Autodesk Inventor part; units mm, degrees
ref_plane "XZ Plane" through (0, 0, 0) normal (0, 1, 0) x (-1, 0, 0)
ref_plane "XY Plane" through (0, 0, 0) normal (0, 0, 1) x (1, 0, 0)
sketch "Sketch1" plane through (0, 0, 0) normal (0, 1, 0) x (-1, 0, 0)
  line L0 (0, 0) -> (0, -60)
  line L1 (0, 0) -> (-50, 0)
  line L2 (-5, -60) -> (-5, -5)
  line L3 (-5, -5) -> (-50, -5)
  line L4 (-47.5, 69.0442) -> (-47.5, -71.5611) construction
  line L5 (-50, 0) -> (-55, 0)
  line L6 (-55, 0) -> (-55, -50)
  line L7 (-55, -50) -> (-75, -50)
  line L8 (-75, -50) -> (-75, -60)
  line L9 (-75, -60) -> (-45, -60)
  line L10 (-5, -60) -> (-21, -60)
  circle A0 centre (-47.5, -73.124) radius 8.5
  line L11 (16.7028, -43.5) -> (-102.7124, -43.5) construction
  line L12 (-45, -26.5) -> (-50, -26.5)
  line L13 (-50, -26.5) -> (-50, -60.5)
  line L14 (-50, -60.5) -> (-45, -60.5)
  line L15 (-45, -60.5) -> (-45, -26.5)
  line L16 (-45, -43.5) -> (-50, -43.5) construction
  line L17 (-21, -60) -> (-21, -67.124)
  line L18 (-21, -67.124) -> (-30, -67.124)
  line L19 (-39, -67.124) -> (-39, -60)
  line L20 (-39, -60) -> (-45, -60) construction
  line L21 (-15.952, -100.4576) -> (-35.952, -100.4576)
  line L22 (-35.952, -108.4576) -> (-15.952, -108.4576)
  line L23 (-15.952, -108.4576) -> (-15.952, -100.4576)
  line L24 (-15.952, -73.124) -> (-76.4965, -73.124) construction
  line L25 (-30, -57.9879) -> (-30, -83.8601) construction
  line L26 (-25.952, -100.4576) -> (-25.952, -108.4576) construction
  line L27 (-45, -31) -> (-50, -31) construction
  line L28 (-50, -31) -> (-50, -56)
  line L29 (-50, -56) -> (-45, -56) construction
  line L30 (-45, -56) -> (-45, -31)
  line L31 (-45, -56) -> (-50, -56)
  line L32 (-45, -65.1391) -> (-45, -56)
  line L33 (-45, -56) -> (-50, -56)
  line L34 (-50, -56) -> (-50, -65)
  line L35 (-50, -65) -> (-45, -65)
  line L36 (-45, -65) -> (-45, -56)
  arc A1 (-35.952, -108.4576) -> (-35.952, -100.4576) centre (-43.452, -104.4576) ccw
  line L37 (-30, -67.124) -> (-39, -67.124)
  point P0 (-47.5, -43.5)
  point P1 (-30, -73.124)
  dimension "d9" = 17
  dimension "d0" = 60
  dimension "d1" = 50
  dimension "d2" = 5
  dimension "d3" = 47.5
  dimension "d4" = 5
  dimension "d5" = 50
  dimension "d6" = 20
  dimension "d7" = 30
  dimension "d10" = 38.5
  dimension "d11" = 5
  dimension "d12" = 34
  dimension "d13" = 20
  dimension "d14" = 8
  dimension "d57" = 25
  dimension "d58" = 4.5
  dimension "d59" = 5
  dimension "d60" = 9
  dimension "d61" = 17
  dimension "d62" = 9
  dimension "d63" = 9
  dimension "d64" = 9
  dimension "d65" = 6
sketch "Sketch2" plane through (0, 0, 0) normal (0, 1, 0) x (-1, 0, 0)
  line L0 (0, 0) -> (-60, 0)
  line L1 (-60, 0) -> (-60, -55)
  line L2 (-57.5, -60) -> (0, -60)
  line L3 (0, -60) -> (0, 0)
  line L4 (-5, -60) -> (-21, -60)
  line L5 (-30, -67.124) -> (-39, -67.124)
  line L6 (-57.5, -67.124) -> (-72, -67.124)
  line L7 (-72, -67.124) -> (-72, -59.124)
  line L8 (-72, -59.124) -> (-60, -59.124)
  line L9 (-60, -59.124) -> (-60, 0)
  line L10 (-57.5, -67.124) -> (-57.5, -60)
  point P0 (-60, -67.124)
  dimension "d16" = 57.5
  dimension "d73" = 8
  dimension "d76" = 12
  dimension "d77" = 60
extrude "Extrusion1" add sketch "Sketch2" along normal blind 20
sketch "Sketch3" plane through (0, 20, 0) normal (0, 1, 0) x (1, 0, 0)
  line L0 (5, 5) -> (55, 5)
  line L1 (55, 5) -> (55, 55)
  line L2 (55, 55) -> (5, 55)
  line L3 (5, 55) -> (5, 5)
  line L4 (0, 0) -> (60, 0)
  line L5 (0, 60) -> (0, 0)
  dimension "d23" = 5
  dimension "d24" = 5
  dimension "d25" = 50
  dimension "d26" = 50
extrude "Extrusion2" cut sketch "Sketch3" against normal blind 10
sketch "Sketch5" plane through (0, 0, 0) normal (0, -1, 0) x (1, 0, 0)
  line L0 (57.5, -60) -> (0, -60)
  line L1 (45, -60.5) -> (45, -26.5)
  line L2 (5, -60) -> (5, -5)
  line L3 (50, -26.5) -> (50, -60.5)
  line L4 (45, -26.5) -> (50, -26.5)
  line L5 (50, -60.5) -> (45, -60.5)
  line L6 (52, -60) -> (52, -24.5)
  line L7 (52, -24.5) -> (43, -24.5)
  line L8 (43, -24.5) -> (43, -60)
  line L9 (52, -60.5) -> (52, -60)
  line L10 (52, -60) -> (43, -60)
  point P0 (80, -60)
  dimension "d30" = 40
  dimension "d31" = 2
extrude "Extrusion3" cut sketch "Sketch5" against normal through all contours L0 L3 L4 L1 L8 L7 L6 | L0 L1 L4 L3
sketch "Sketch6" plane through (0, 0, 0) normal (0, 0, 1) x (1, 0, 0)
  line L0 (0, 20) -> (60, 20)
  line L1 (47.5, 0) -> (47.5, 20) construction
  circle A0 centre (47.5, 10) radius 7
  point P0 (47.5, 0)
  dimension "d34" = 14
extrude "Extrusion4" add sketch "Sketch6" along normal blind 25
ref_plane "Work Plane1" through (54.5, 10, 0) normal (1, 0, 0) x (0, 1, 0)
sketch "Sketch7" plane through (54.5, 10, 0) normal (1, 0, 0) x (0, 1, 0)
  line L0 (7, 25) -> (-7, 25)
  line L1 (0, 25) -> (0, 0) construction
  point P0 (-10, 0)
  point P1 (0, 17)
  dimension "d37" = 8
hole "Hole1" at (54.5, 10, 17) direction (-1, 0, 0) diameter 5 end through all
sketch "Sketch8" plane through (0, 10, 0) normal (0, 1, 0) x (1, 0, 0)
  line L0 (36, 11.5) -> (39, 11.5)
  line L1 (39, 11.5) -> (39, 43.5)
  line L2 (39, 43.5) -> (36, 43.5)
  line L3 (36, 43.5) -> (36, 11.5)
  line L4 (45, 60.5) -> (45, 26.5)
  line L5 (-16.7028, 43.5) -> (102.7124, 43.5) construction
  point P0 (0, 0)
  point P1 (47.5, 43.5)
  dimension "d45" = 6
  dimension "d46" = 32
  dimension "d47" = 3
extrude "Extrusion5" cut sketch "Sketch8" against normal blind 4
sketch "Sketch9" plane through (0, 10, 0) normal (0, 1, 0) x (1, 0, 0)
  line L0 (36, 43.5) -> (39, 43.5)
  line L1 (5, 5) -> (5, 55)
  line L2 (8, 18.5) -> (5, 18.5)
  line L3 (5, 18.5) -> (5, 38.5)
  line L4 (5, 38.5) -> (8, 38.5)
  line L5 (8, 38.5) -> (8, 18.5)
  point P0 (0, 0)
  dimension "d50" = 3
  dimension "d51" = 5
  dimension "d52" = 20
extrude "Extrusion6" add sketch "Sketch9" along normal up to surface (10 mm away)
fillet "Fillet1" radius 0.6 4 edges at (5, 15, -38.5) (8, 15, -38.5) (8, 15, -18.5) (5, 15, -18.5)
fillet "Fillet2" radius 1 2 edges at (43, 5, -24.5) (52, 5, -24.5)
sketch "Sketch10" plane through (0, 0, 0) normal (0, -1, 0) x (1, 0, 0)
  line L0 (43, -60) -> (0, -60)
  line L1 (39, -67.124) -> (39, -60)
  line L2 (30, -67.124) -> (39, -67.124)
  line L3 (21, -60) -> (21, -67.124)
  line L4 (21, -67.124) -> (30, -67.124)
  line L5 (39, -60) -> (39, -67.124)
  line L6 (21, -67.124) -> (39, -67.124)
  line L7 (21, -67.124) -> (21, -60)
  point P0 (80, -60)
extrude "Extrusion7" add sketch "Sketch10" against normal up to surface (20 mm away)
sketch "Sketch11" plane through (0, 20, 0) normal (0, 1, 0) x (1, 0, 0)
  line L0 (39, 67.124) -> (39, 60)
  line L1 (21, 67.124) -> (39, 67.124)
  line L2 (21, 60) -> (21, 67.124)
  line L3 (5, 55) -> (55, 55)
  line L4 (25.5, 55) -> (34.5, 55)
  line L5 (34.5, 55) -> (34.5, 61.124)
  line L6 (34.5, 61.124) -> (25.5, 61.124)
  line L7 (25.5, 61.124) -> (25.5, 55)
  dimension "d68" = 6
  dimension "d69" = 4.5
  dimension "d70" = 4.5
extrude "Extrusion8" cut sketch "Sketch11" against normal up to surface (10 mm away)
sketch "Sketch12" plane through (0, 20, 0) normal (0, 1, 0) x (1, 0, 0)
  line L0 (34.5, 61.124) -> (34.5, 55)
  line L1 (34.5, 55) -> (43, 55)
  line L2 (43, 55) -> (43, 60)
  line L3 (43, 60) -> (39, 60)
  line L4 (39, 67.124) -> (39, 60)
  line L5 (21, 67.124) -> (39, 67.124)
  line L6 (21, 60) -> (21, 67.124)
  line L7 (21, 60) -> (0, 60)
  line L8 (0, 60) -> (0, 0)
  line L9 (0, 0) -> (60, 0)
  line L10 (60, 0) -> (60, 59.124)
  line L11 (60, 59.124) -> (72, 59.124)
  line L12 (72, 59.124) -> (72, 67.124)
  line L13 (72, 67.124) -> (57.5, 67.124)
  line L14 (57.5, 67.124) -> (57.5, 60)
  line L15 (57.5, 60) -> (52, 60)
  line L16 (52, 60) -> (52, 55)
  line L17 (52, 55) -> (55, 55)
  line L18 (55, 55) -> (55, 5)
  line L19 (55, 5) -> (5, 5)
  line L20 (5, 5) -> (5, 17.9)
  arc A0 (5.6, 18.5) -> (5, 17.9) centre (5.6, 17.9) ccw
  line L21 (7.4, 18.5) -> (5.6, 18.5)
  arc A1 (7.4, 18.5) -> (8, 19.1) centre (7.4, 19.1) ccw
  line L22 (8, 37.9) -> (8, 19.1)
  arc A2 (8, 37.9) -> (7.4, 38.5) centre (7.4, 37.9) ccw
  line L23 (5.6, 38.5) -> (7.4, 38.5)
  arc A3 (5, 39.1) -> (5.6, 38.5) centre (5.6, 39.1) ccw
  line L24 (5, 39.1) -> (5, 55)
  line L25 (5, 55) -> (25.5, 55)
  line L26 (25.5, 55) -> (25.5, 61.124)
  line L27 (25.5, 61.124) -> (34.5, 61.124)
  line L28 (65, 73.0401) -> (65, 59.124)
  circle A4 centre (47.5, 73.124) radius 8.5
  point P0 (60, 52.124)
  point P1 (60, 57.124)
  point P2 (62, 59.124)
  dimension "d74" = 9
sketch "Sketch13" plane through (0, 0, 0) normal (0, -1, 0) x (1, 0, 0)
  line L0 (60, 0) -> (60, -59.124)
  line L1 (72, -59.124) -> (60, -24.124)
  line L2 (60, 0) -> (60, -59.124)
  line L3 (60, -59.124) -> (60, -24.124)
  line L4 (72, -59.124) -> (60, -59.124)
  dimension "d78" = 35
extrude "Extrusion9" add sketch "Sketch13" against normal blind 5
equation "\"d70\" = d69"
properties part number "Housing"
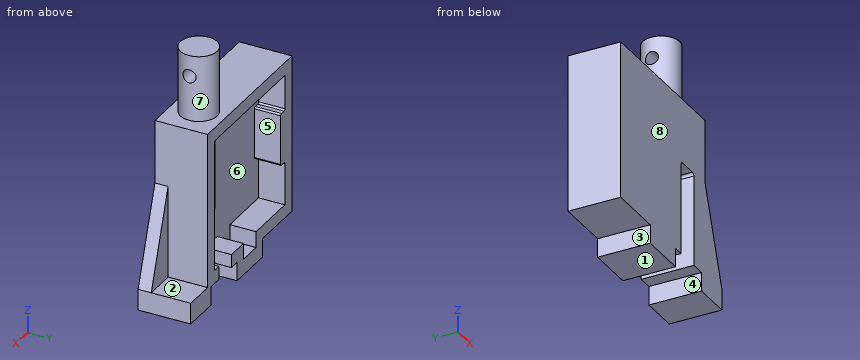
Can you work these out from the model? Positions are in its coordinate system, mm. Face numbers are marked on the shaded views. A direction names the side the tool comes from. Coordinates: 2 decimals unless noted, no trailing zeros. Loops run counter-clockwise (first coordinate to the right, second up) from the corner with the lowest first, then second, coordinate; pieces in that order, holes last. Notation, with made-up numbers: (-31, 18.5) -> (7, 18.5) arc R27 ccw to (7, 35.5) -> close; hole circle Ø4 at (34.5, 2.5). An arc over 180 degrees is marked (long way). Put each result on its own line as item: value. Start each with the question number.
Q1. If I drill on line 1 (X direction, y = 14, z = -24); line 2 (X direction, y = 8.5, z = -58); line 3 (Z direction, x = 38.5, y = 17.75), over which ranges is the centre line in solid material (lowest first)? Write a range as [from, to].
Q2. I want a section at C-C (z = -48). Write out the boundary of the cut face in (x, y), plus the area to 3 significant figures.
Q3. For the marked faces 1, 2, 3, 4 and 5, which set-ups out of +Z, -Z, +X, -X, +Y, -Y let a thin tool reach every point of the face, with its end or its side?
Q4. I'm going to push flat-ended pins straight in: P1, Ø1.6, axis at x = 55.5, y = 12.5, coming from the -Z side; P2, Ø3, axis at y = 10, z = -8, coming from the +X side; P3, Ø1, axis at y = 2.5, z = -56, coming from the +X side. Where does each tip first touch, or does it pass through?
Q5. I want a section at D-D (x = 12). Write out the boundary of the cut face in (y, z), plus the area to 3 significant figures.
Q6. Thinking about a two-plate mould opening in X: for the marked faces 6, 7 and 8, which applies, pulls with the +X half, pulls with the -X half, needs draft (parallel to the pull), parting line crosses it, or undercut?
Q7. I want a section at B-B (z = -10). Write out the boundary of the cut face in (x, y), plus the area to 3 significant figures.
Q8. I want a section at A-A (x = 47.5). Write out the boundary of the cut face in (y, z).
Taken from the geometry:
1. line 1: x = [0, 8], [55, 60]
1. line 2: x = [0, 43], [52, 60]
1. line 3: z = [-67.12, -55], [-5, 0]
2. outline: (0, 0) -> (43, 0) -> (43, 10) -> (5, 10) -> (5, 20) -> (0, 20) -> close; (52, 0) -> (68.19, 0) -> (68.19, 5) -> (60, 5) -> (60, 20) -> (55, 20) -> (55, 10) -> (52, 10) -> close
2. area: 651 mm2
3. face 1: -Z, +X, -X, +Y, -Y
3. face 2: +Z, +X, +Y
3. face 3: -Z, -X, +Y, -Y
3. face 4: -Z, +Y, -Y
3. face 5: +Y
4. P1: stops at z = -60
4. P2: stops at x = 60
4. P3: stops at x = 71.1
5. outline: (0, -60) -> (20, -60) -> (20, -55) -> (10, -55) -> (10, -5) -> (20, -5) -> (20, 0) -> (0, 0) -> close
5. area: 700 mm2
6. face 6: undercut
6. face 7: parting line crosses it
6. face 8: needs draft
7. outline: (0, 0) -> (60, 0) -> (60, 20) -> (55, 20) -> (55, 10) -> (5, 10) -> (5, 20) -> (0, 20) -> close
7. area: 700 mm2
8. outline: (0, -24.5) -> (10, -24.5) -> (10, -5) -> (20, -5) -> (20, 0) -> (17, 0) -> (17, 25) -> (3, 25) -> (3, 0) -> (0, 0) -> close; hole circle Ø5 at (10, 17)
